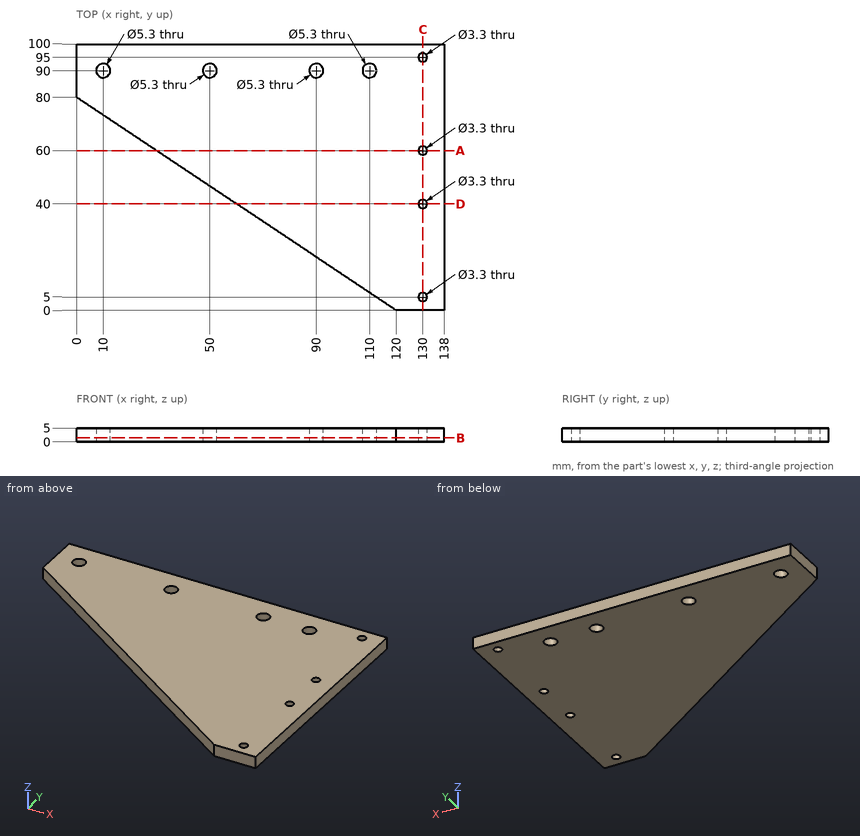
Print and shaded views of the part. All mm, measured from the part's lowest x, y and z. Coordinates: 2 decimals unless noted, no trailing zeros. Order: outer loops, then holes, each group sorted by start corner. A loop starts at its lowest first (then second) coordinate and runs counter-clockwise, first axis right, second up. Notation, with made-up numbers: M 36.25,-2 L 94.25,-2 A13 cw 94.25,10 Z; hole C 3,58 d3. An arc over 180 degrees is marked long. Answer as CSV lines item,"result".
1) Drill centre lines: L1, parallel to Y at x = 130, z = 3.85; L2, parallel to X at y = 95, z = 3.3; L3, parallel to Y at x = 111, z = 3.9. Where is each one in solid material? Low to high. Write a range as from..to.
Verdict:
L1,"0..3.35, 6.65..38.35, 41.65..58.35, 61.65..93.35, 96.65..100"
L2,"0..128.35, 131.65..138"
L3,"6..87.55, 92.45..100"
2) Flat gauge pins, fed straight in: P1, Ø5.5, axis at x = 130, y = 40, coming from the -Z side; P2, Ø3, axis at x = 130, y = 5, coming from the +Z side. Where does each tip first touch, or does it go through?
Verdict:
P1,"z = 0"
P2,"through"
3) Cut at C-C (x = 130). List the corners of the cut face in (y, z), then the cut area to 3 significant figures.
Verdict:
outline,"M 0,0 L 3.35,0 L 3.35,5 L 0,5 Z; M 6.65,0 L 38.35,0 L 38.35,5 L 6.65,5 Z; M 41.65,0 L 58.35,0 L 58.35,5 L 41.65,5 Z; M 61.65,0 L 93.35,0 L 93.35,5 L 61.65,5 Z; M 96.65,0 L 100,0 L 100,5 L 96.65,5 Z"
area,"434 mm2"
4) Cut at B-B (z = 1.4). Give the number of separate pieces and of enclosed holes in the cut face, then the cut area to 3 significant figures.
Verdict:
separate pieces,"1"
enclosed holes,"8"
area,"8,880 mm2"
5) Cut at A-A (y = 60). List the corners of the cut face in (x, z), then the cut area to 4 significant figures.
Verdict:
outline,"M 30,0 L 128.35,0 L 128.35,5 L 30,5 Z; M 131.65,0 L 138,0 L 138,5 L 131.65,5 Z"
area,"523.5 mm2"
6) Cut at D-D (y = 40). List the corners of the cut face in (x, z), then the cut area to 4 significant figures.
Verdict:
outline,"M 60,0 L 128.35,0 L 128.35,5 L 60,5 Z; M 131.65,0 L 138,0 L 138,5 L 131.65,5 Z"
area,"373.5 mm2"
